```python
from build123d import *

# Parameters (mm, degrees)
SKETCH1_R              = 11
SKETCH1_R_2            = 10
SKETCH1_R_3            = 1.25
SKETCH1_R_4            = 1.5
BOSS_EXTRUDE1_DEPTH    = 6
SKETCH2_W              = 15
SKETCH2_H              = 22
BOSS_EXTRUDE2_DEPTH    = 6
CHAMFER1_SIZE          = 1
SKETCH3_R              = 1
CUT_EXTRUDE1_DEPTH     = 159.031622749
FILLET1_R              = 10
MOVE_FACE1_OUTLINE_R   = 11
MOVE_FACE1_OUTLINE_R_2 = 10.92
MOVE_FACE1_OUTLINE_R_3 = 10
MOVE_FACE1_OUTLINE_R_4 = 9.92
MOVE_FACE1_OUTLINE_R_5 = 1.25
MOVE_FACE1_OUTLINE_R_6 = 1.17
MOVE_FACE1_OUTLINE_R_7 = 1.5
MOVE_FACE1_OUTLINE_R_8 = 1.42
MOVE_FACE1_DEPTH       = 6


# Read off the part's stored shape, not the designer's step: Move Face1
with BuildPart() as part:
    # Sketch1 → Boss-Extrude1 (new body)
    with BuildSketch(Plane.XY):
        with BuildLine():
            Line((-40.498784978, 0), (0, 0))
            Line((0, 0), (0, 75))
            ThreePointArc((0, 75), (-37.5, 112.5), (-75, 75))
            Line((-75, 75), (-75, 55))
            Line((-75, 55), (-83.323029145, 55))
            ThreePointArc((-83.323029145, 55), (-110.823029145, 27.5), (-83.323029145, 0))
            Line((-83.323029145, 0), (-40.498784978, 0))
        make_face()
        with Locations((-83.323029145, 27.5)):
            Circle(SKETCH1_R, mode=Mode.SUBTRACT)
        with Locations((-37.5, 75)):
            Circle(SKETCH1_R_2, mode=Mode.SUBTRACT)
        with Locations((-83.323029145, 50.5)):
            Circle(SKETCH1_R_3, mode=Mode.SUBTRACT)
        with Locations((-67.059573177, 43.763455967)):
            Circle(SKETCH1_R_4, mode=Mode.SUBTRACT)
        with Locations((-37.5, 102.5)):
            Circle(SKETCH1_R_3, mode=Mode.SUBTRACT)
        with Locations((-10, 75)):
            Circle(SKETCH1_R_3, mode=Mode.SUBTRACT)
        with Locations((-37.5, 47.5)):
            Circle(SKETCH1_R_3, mode=Mode.SUBTRACT)
        with Locations((-65, 75)):
            Circle(SKETCH1_R_3, mode=Mode.SUBTRACT)
        with Locations((-56.945436483, 94.445436483)):
            Circle(SKETCH1_R_4, mode=Mode.SUBTRACT)
        with Locations((-60.323029145, 27.5)):
            Circle(SKETCH1_R_3, mode=Mode.SUBTRACT)
        with Locations((-67.059573177, 11.236544033)):
            Circle(SKETCH1_R_4, mode=Mode.SUBTRACT)
        with Locations((-83.323029145, 4.5)):
            Circle(SKETCH1_R_3, mode=Mode.SUBTRACT)
        with Locations((-18.054563517, 94.445436483)):
            Circle(SKETCH1_R_4, mode=Mode.SUBTRACT)
        with Locations((-18.054563517, 55.554563517)):
            Circle(SKETCH1_R_4, mode=Mode.SUBTRACT)
        with Locations((-56.945436483, 55.554563517)):
            Circle(SKETCH1_R_4, mode=Mode.SUBTRACT)
        with Locations((-37.5, 88)):
            Circle(SKETCH1_R_3, mode=Mode.SUBTRACT)
        with Locations((-50.5, 75)):
            Circle(SKETCH1_R_3, mode=Mode.SUBTRACT)
        with Locations((-37.5, 62)):
            Circle(SKETCH1_R_3, mode=Mode.SUBTRACT)
        with Locations((-24.5, 75)):
            Circle(SKETCH1_R_3, mode=Mode.SUBTRACT)
    extrude(amount=BOSS_EXTRUDE1_DEPTH)

    # Sketch2 → Boss-Extrude2 (add)
    with BuildSketch(Plane(origin=(0, 0, 0), x_dir=(-1, 0, 0), z_dir=(0, 0, -1))):
        with Locations((7.5, -11)):
            Rectangle(SKETCH2_W, SKETCH2_H)
        with Locations((37.5, -11)):
            Rectangle(SKETCH2_W, SKETCH2_H)
        with Locations((67.5, -11)):
            Rectangle(SKETCH2_W, SKETCH2_H)
    extrude(amount=-BOSS_EXTRUDE2_DEPTH)

    # Chamfer1
    chamfer1_edges = [part.edges().sort_by_distance(p)[0] for p in [
        (0, -22, 3),
        (-15, -22, 3),
        (-30, -22, 3),
        (-45, -22, 3),
        (-60, -22, 3),
        (-75, -22, 3),
    ]]
    chamfer(chamfer1_edges, length=CHAMFER1_SIZE)

    # Sketch3 → Cut-Extrude1 (cut, through all)
    with BuildSketch(Plane.XY.offset(6)):
        with Locations((-75, 0)):
            Circle(SKETCH3_R)
        with Locations((-60, 0)):
            Circle(SKETCH3_R)
        with Locations((-45, 0)):
            Circle(SKETCH3_R)
        with Locations((-30, 0)):
            Circle(SKETCH3_R)
        with Locations((-15, 0)):
            Circle(SKETCH3_R)
    extrude(amount=-CUT_EXTRUDE1_DEPTH, mode=Mode.SUBTRACT)

    # Fillet1
    fillet1_edges = [part.edges().sort_by_distance(p)[0] for p in [
        (-75, 55, 3),
    ]]
    fillet(fillet1_edges, radius=FILLET1_R)

    # Move Face1 outline → Move Face1 (add)
    # profile 1 of 25: a face of its own
    with BuildSketch(Plane.XY):
        with BuildLine():
            Line((-59.003205136, -0.08), (-45.996794864, -0.08))
            ThreePointArc((-45.996794864, -0.08), (-45.999198395, -0.04003209), (-46, 0))
            Line((-46, 0), (-59, 0))
            ThreePointArc((-59, 0), (-59.000801605, -0.04003209), (-59.003205136, -0.08))
        make_face()
    # profile 2 of 25: a face of its own
    with BuildSketch(Plane.XY):
        with BuildLine():
            Line((-45, -21), (-45, -1))
            ThreePointArc((-45, -1), (-45.04003209, -0.999198395), (-45.08, -0.996794864))
            Line((-45.08, -0.996794864), (-45.08, -21.033137085))
            Line((-45.08, -21.033137085), (-44.033137085, -22.08))
            Line((-44.033137085, -22.08), (-30.966862915, -22.08))
            Line((-30.966862915, -22.08), (-29.92, -21.033137085))
            Line((-29.92, -21.033137085), (-29.92, -0.996794864))
            ThreePointArc((-29.92, -0.996794864), (-29.95996791, -0.999198395), (-30, -1))
            Line((-30, -1), (-30, -21))
            Line((-30, -21), (-31, -22))
            Line((-31, -22), (-44, -22))
            Line((-44, -22), (-45, -21))
        make_face()
    # profile 3 of 25: a face of its own
    with BuildSketch(Plane.XY):
        with BuildLine():
            ThreePointArc((-59.92, -0.996794864), (-59.95996791, -0.999198395), (-60, -1))
            Line((-60, -1), (-60, -21))
            Line((-60, -21), (-61, -22))
            Line((-61, -22), (-74, -22))
            Line((-74, -22), (-73.92, -22.08))
            Line((-73.92, -22.08), (-60.966862915, -22.08))
            Line((-60.966862915, -22.08), (-59.92, -21.033137085))
            Line((-59.92, -21.033137085), (-59.92, -0.996794864))
        make_face()
    # profile 4 of 25: a face of its own
    with BuildSketch(Plane.XY):
        with BuildLine():
            Line((-75.08, -20.92), (-75, -21))
            Line((-75, -21), (-75, -1))
            ThreePointArc((-75, -1), (-75.04003209, -0.999198395), (-75.08, -0.996794864))
            Line((-75.08, -0.996794864), (-75.08, -20.92))
        make_face()
    # profile 5 of 25: a face of its own
    with BuildSketch(Plane.XY):
        with BuildLine():
            Line((-16, 0), (-29, 0))
            ThreePointArc((-29, 0), (-29.000801605, -0.04003209), (-29.003205136, -0.08))
            Line((-29.003205136, -0.08), (-15.996794864, -0.08))
            ThreePointArc((-15.996794864, -0.08), (-15.999198395, -0.04003209), (-16, 0))
        make_face()
    # profile 6 of 25: a face of its own
    with BuildSketch(Plane.XY):
        with BuildLine():
            Line((-85.422171827, 0), (-83.323029145, 0))
            ThreePointArc((-83.323029145, 0), (-110.816150501, 26.884956844), (-84.552807772, 54.972488867))
            ThreePointArc((-84.552807772, 54.972488867), (-77.772555006, 58.051331596), (-75, 64.962484818))
            Line((-75, 64.962484818), (-75, 75))
            ThreePointArc((-75, 75), (-37.5, 112.5), (0, 75))
            Line((0, 75), (0, -21))
            Line((0, -21), (-1, -22))
            Line((-1, -22), (-14, -22))
            Line((-14, -22), (-15, -21))
            Line((-15, -21), (-15, -1))
            ThreePointArc((-15, -1), (-15.04003209, -0.999198395), (-15.08, -0.996794864))
            Line((-15.08, -0.996794864), (-15.08, -21.033137085))
            Line((-15.08, -21.033137085), (-14.033137085, -22.08))
            Line((-14.033137085, -22.08), (-0.966862915, -22.08))
            Line((-0.966862915, -22.08), (0.08, -21.033137085))
            Line((0.08, -21.033137085), (0.08, 75))
            ThreePointArc((0.08, 75), (-37.5, 112.58), (-75.08, 75))
            Line((-75.08, 75), (-75.08, 64.962484818))
            ThreePointArc((-75.08, 64.962484818), (-77.830374566, 58.106620822), (-84.55638531, 55.052408834))
            ThreePointArc((-84.55638531, 55.052408834), (-110.899619158, 27.933685652), (-85.422171827, 0))
        make_face()
    # profile 7 of 25: a face of its own
    with BuildSketch(Plane.XY):
        with Locations((-83.323029145, 27.5)):
            Circle(MOVE_FACE1_OUTLINE_R)
        with Locations((-83.323029145, 27.5)):
            Circle(MOVE_FACE1_OUTLINE_R_2, mode=Mode.SUBTRACT)
    # profile 8 of 25: a face of its own
    with BuildSketch(Plane.XY):
        with Locations((-37.5, 75)):
            Circle(MOVE_FACE1_OUTLINE_R_3)
        with Locations((-37.5, 75)):
            Circle(MOVE_FACE1_OUTLINE_R_4, mode=Mode.SUBTRACT)
    # profile 9 of 25: a face of its own
    with BuildSketch(Plane.XY):
        with Locations((-83.323029145, 50.5)):
            Circle(MOVE_FACE1_OUTLINE_R_5)
        with Locations((-83.323029145, 50.5)):
            Circle(MOVE_FACE1_OUTLINE_R_6, mode=Mode.SUBTRACT)
    # profile 10 of 25: a face of its own
    with BuildSketch(Plane.XY):
        with Locations((-67.059573177, 43.763455967)):
            Circle(MOVE_FACE1_OUTLINE_R_7)
        with Locations((-67.059573177, 43.763455967)):
            Circle(MOVE_FACE1_OUTLINE_R_8, mode=Mode.SUBTRACT)
    # profile 11 of 25: a face of its own
    with BuildSketch(Plane.XY):
        with Locations((-37.5, 102.5)):
            Circle(MOVE_FACE1_OUTLINE_R_5)
        with Locations((-37.5, 102.5)):
            Circle(MOVE_FACE1_OUTLINE_R_6, mode=Mode.SUBTRACT)
    # profile 12 of 25: a face of its own
    with BuildSketch(Plane.XY):
        with Locations((-10, 75)):
            Circle(MOVE_FACE1_OUTLINE_R_5)
        with Locations((-10, 75)):
            Circle(MOVE_FACE1_OUTLINE_R_6, mode=Mode.SUBTRACT)
    # profile 13 of 25: a face of its own
    with BuildSketch(Plane.XY):
        with Locations((-37.5, 47.5)):
            Circle(MOVE_FACE1_OUTLINE_R_5)
        with Locations((-37.5, 47.5)):
            Circle(MOVE_FACE1_OUTLINE_R_6, mode=Mode.SUBTRACT)
    # profile 14 of 25: a face of its own
    with BuildSketch(Plane.XY):
        with Locations((-65, 75)):
            Circle(MOVE_FACE1_OUTLINE_R_5)
        with Locations((-65, 75)):
            Circle(MOVE_FACE1_OUTLINE_R_6, mode=Mode.SUBTRACT)
    # profile 15 of 25: a face of its own
    with BuildSketch(Plane.XY):
        with Locations((-56.945436483, 94.445436483)):
            Circle(MOVE_FACE1_OUTLINE_R_7)
        with Locations((-56.945436483, 94.445436483)):
            Circle(MOVE_FACE1_OUTLINE_R_8, mode=Mode.SUBTRACT)
    # profile 16 of 25: a face of its own
    with BuildSketch(Plane.XY):
        with Locations((-37.5, 88)):
            Circle(MOVE_FACE1_OUTLINE_R_5)
        with Locations((-37.5, 88)):
            Circle(MOVE_FACE1_OUTLINE_R_6, mode=Mode.SUBTRACT)
    # profile 17 of 25: a face of its own
    with BuildSketch(Plane.XY):
        with Locations((-60.323029145, 27.5)):
            Circle(MOVE_FACE1_OUTLINE_R_5)
        with Locations((-60.323029145, 27.5)):
            Circle(MOVE_FACE1_OUTLINE_R_6, mode=Mode.SUBTRACT)
    # profile 18 of 25: a face of its own
    with BuildSketch(Plane.XY):
        with Locations((-67.059573177, 11.236544033)):
            Circle(MOVE_FACE1_OUTLINE_R_7)
        with Locations((-67.059573177, 11.236544033)):
            Circle(MOVE_FACE1_OUTLINE_R_8, mode=Mode.SUBTRACT)
    # profile 19 of 25: a face of its own
    with BuildSketch(Plane.XY):
        with Locations((-83.323029145, 4.5)):
            Circle(MOVE_FACE1_OUTLINE_R_5)
        with Locations((-83.323029145, 4.5)):
            Circle(MOVE_FACE1_OUTLINE_R_6, mode=Mode.SUBTRACT)
    # profile 20 of 25: a face of its own
    with BuildSketch(Plane.XY):
        with Locations((-18.054563517, 94.445436483)):
            Circle(MOVE_FACE1_OUTLINE_R_7)
        with Locations((-18.054563517, 94.445436483)):
            Circle(MOVE_FACE1_OUTLINE_R_8, mode=Mode.SUBTRACT)
    # profile 21 of 25: a face of its own
    with BuildSketch(Plane.XY):
        with Locations((-18.054563517, 55.554563517)):
            Circle(MOVE_FACE1_OUTLINE_R_7)
        with Locations((-18.054563517, 55.554563517)):
            Circle(MOVE_FACE1_OUTLINE_R_8, mode=Mode.SUBTRACT)
    # profile 22 of 25: a face of its own
    with BuildSketch(Plane.XY):
        with Locations((-56.945436483, 55.554563517)):
            Circle(MOVE_FACE1_OUTLINE_R_7)
        with Locations((-56.945436483, 55.554563517)):
            Circle(MOVE_FACE1_OUTLINE_R_8, mode=Mode.SUBTRACT)
    # profile 23 of 25: a face of its own
    with BuildSketch(Plane.XY):
        with Locations((-50.5, 75)):
            Circle(MOVE_FACE1_OUTLINE_R_5)
        with Locations((-50.5, 75)):
            Circle(MOVE_FACE1_OUTLINE_R_6, mode=Mode.SUBTRACT)
    # profile 24 of 25: a face of its own
    with BuildSketch(Plane.XY):
        with Locations((-37.5, 62)):
            Circle(MOVE_FACE1_OUTLINE_R_5)
        with Locations((-37.5, 62)):
            Circle(MOVE_FACE1_OUTLINE_R_6, mode=Mode.SUBTRACT)
    # profile 25 of 25: a face of its own
    with BuildSketch(Plane.XY):
        with Locations((-24.5, 75)):
            Circle(MOVE_FACE1_OUTLINE_R_5)
        with Locations((-24.5, 75)):
            Circle(MOVE_FACE1_OUTLINE_R_6, mode=Mode.SUBTRACT)
    extrude(amount=MOVE_FACE1_DEPTH)


solid = part.part
```
Input: part model. Units: mm. Frame: model coordinates. A direction names the side the tool comes from. Coordinates: 2 decimals unless noted, no trailing zeros. Write each loop counter-clockwise with the first axis right and the second up, starting at its lowest first coordinate (ties: lowest second). Pieces come first, ordered by that corner, then holes. Notation, with made-up numbers: M -34.5,74.5 L 4.5,74.5 A33 ccw 4.5,106.5 Z; hole C -29.75,20 d9. An arc over 180 degrees is marked long. Use one line per item in the form item = value.
Q1. Material intervals for probe 1 along Y at (x, z) = (-37.5, 2.25); probe 2 along X at (y, z) = (-4, 1.45); probe 3 along X at (y, z) = (64.5, 1.3), sorted ascending. Write a range as from..to.
Answer below:
probe_1 = -22.08..46.33, 48.67..60.83, 63.17..65.08, 84.92..86.83, 89.17..101.33, 103.67..112.58
probe_2 = -75.08..-59.92, -45.08..-29.92, -15.08..0.08
probe_3 = -75.09..0.08
Q2. Section D-D (y = 15). Return loops of the section in (x, z).
Answer below:
outline = M -107.91,0 L 0.08,0 L 0.08,6 L -107.91,6 Z
Q3. First-contact query: pin 1 (1.8 mm diameter, centred on x = -23.5, z = 2.5, fed in from -Y); pin 2 (1.8 mm diameter, centred on y = -14, z = 2.5, fed in from -X); pin 3 (2.5 mm diameter, centred on x = -56.95, y = 55.55, fed in from +Z); pin 4 (1 mm diameter, centred on x = -17.5, z = 2, fed in from +Y). Flat tips, straight axial feed; report the tip coordinate or a pass-through.
Answer below:
pin_1 = -0.08
pin_2 = -75.08
pin_3 = through
pin_4 = 107.12
Q4. Draft query along Y for faces 1 (the face through (-91.99, 20.86, 2.96)), 2 (the face through (-77.76, 58.18, 2.96)), 3 (the face through (-68, -22.08, 3)), 4 (the face through (-55.59, 55.98, 2.96)). Return one class per face: released by +Y, released by -Y, zero draft, split by the parting line, or undercut.
Answer below:
face_1 = undercut
face_2 = released by +Y
face_3 = released by -Y
face_4 = undercut
Q5. Section A-A (y = -8). Return loops of the section in (x, z), plus the area to 3 significant figures.
Answer below:
outline = M -75.08,0 L -59.92,0 L -59.92,6 L -75.08,6 Z; M -45.08,0 L -29.92,0 L -29.92,6 L -45.08,6 Z; M -15.08,0 L 0.08,0 L 0.08,6 L -15.08,6 Z
area = 273 mm²
Q6. Set-up query: faces 5 (the face through (-81, 0, 3)), 6 (the face through (-53, -0.08, 3)), 7 (the face through (-17.399, 54.295, 2.958)). Return all of +Z, -Z, +X, -X, +Y, -Y with unobstructed straight access to the full face (end or side cutting, diameter ignored); none if empty.
Answer below:
face_5 = +Z, -Z, -X, -Y
face_6 = +Z, -Z, -Y
face_7 = +Z, -Z
Q7. Section C-C (z = 4.4). Count the separate pieces of the cut face and the enclosed holes in it, plus the area to 3 significant figures.
Answer below:
separate_pieces = 1
enclosed_holes = 19
area = 9,750 mm²
Q8. Section B-B (x = -42). Return loops of the section in (y, z), plus the area to 3 significant figures.
Answer below:
outline = M -22.08,0 L 66.16,0 L 66.16,6 L -22.08,6 Z; M 83.84,0 L 112.31,0 L 112.31,6 L 83.84,6 Z
area = 700 mm²
